Input: dimensioned drawing with shaded views. Units: mm. Origin: part minimum x, y, z. A direction names the side the tool comes from. Round coordinates to 2 decimals unless told otherwise and drop trailing zeros. Write each loop counter-clockwise with the first axis right and the second up, starting at its lowest first coordinate (ties: lowest second). Pieces come first, ordered by that corner, then holes. Notation, with made-up numbers: M 87,-34.5 L 102,-34.5 A29 ccw 102,-5.5 Z; hole C -36,11.5 d4. An arc over 180 degrees is marked long. Answer in a Markdown table with one row per item. Add a question column.
Item 1: Contact query for flat-ended pins moving along their axis: pin 1 (12 mm diameter, centred on x = 569, z = 661.5, fed in from -Y); pin 2 (12 mm diameter, centred on y = 489, z = 665.5, fed in from +X). Output: stop coordinate, or through.
Item 2: Cut plane D-D on z = 83. Return loops of the section in (x, y), and give its area (3 significant figures).
Item 3: Set-up query: the marked faces 1, 2, 3 and 4. Return all of +Z, -Z, +X, -X, +Y, -Y with unobstructed straight access to the full face (end or side cutting, diameter ignored); none if empty.
Item 4: Cut plane A-A on y = 268. Return loops of the section in (x, z) (1 decimal).
Item 5: Material intervals for probe 1 along Z at (x, y) = (132, 424.5) (1 decimal); probe 2 along Y at (x, z) = (1610, 397.5); probe 3 along X at (y, z) = (741, 596.5), sorted ascending.
Item 6: Cut plane B-B on x = 141.5. Return loops of the section in (y, z) (1 decimal).
Item 7: Cut plane C-C on y = 79. Return loops of the section in (x, z) (1 decimal), and give its area (3 significant figures).
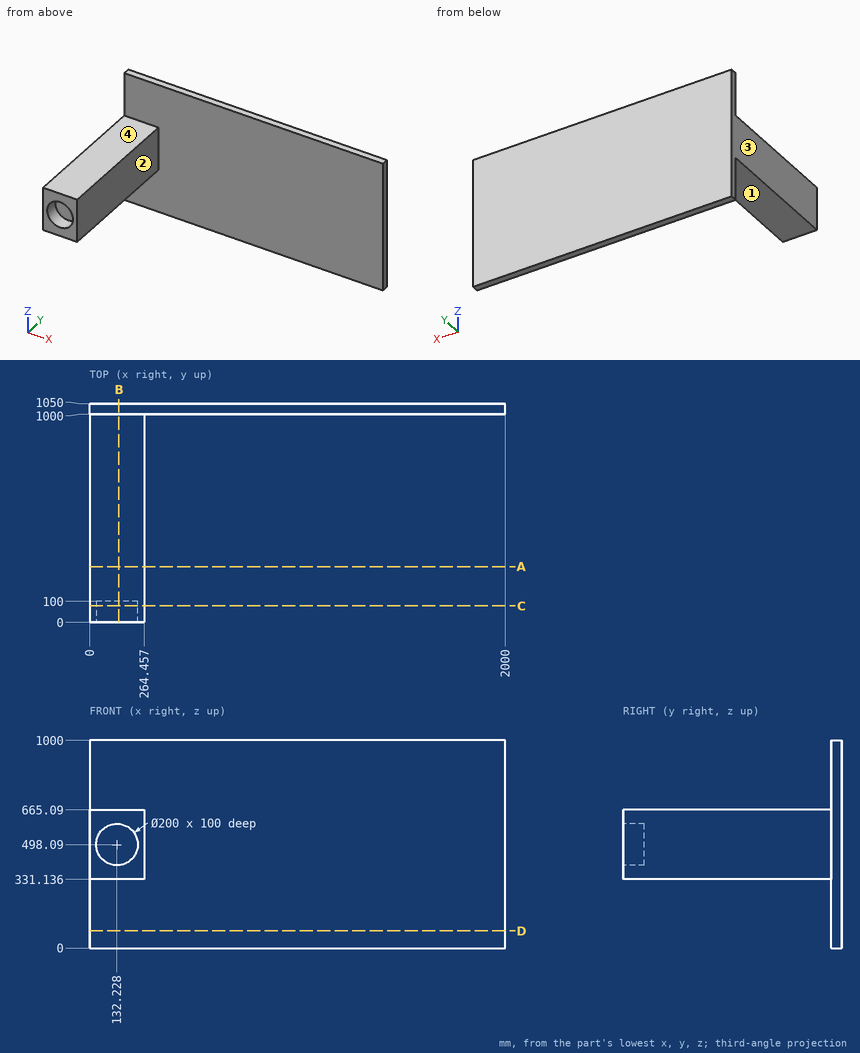
Results below:
| question | item | result |
|---|---|---|
| 1 | pin 1 | y = 1000 |
| 1 | pin 2 | x = 264.46 |
| 2 | outline | M 0,1000 L 2000,1000 L 2000,1050 L 0,1050 Z |
| 2 | area | 100,000 mm2 |
| 3 | face 1 | -Z, +X, -X, -Y |
| 3 | face 2 | +Z, -Z, +X, -Y |
| 3 | face 3 | +Z, -Z, -X, +Y, -Y |
| 3 | face 4 | +Z, +X, -X, -Y |
| 4 | outline | M 0,331.1 L 264.5,331.1 L 264.5,665.1 L 0,665.1 Z |
| 5 | probe 1 | 331.1 to 665.1 |
| 5 | probe 2 | 1000 to 1050 |
| 5 | probe 3 | 0 to 264.46 |
| 6 | outline | M 0,331.1 L 1000,331.1 L 1000,0 L 1050,0 L 1050,1000 L 1000,1000 L 1000,665.1 L 0,665.1 L 0,597.7 L 100,597.7 L 100,398.5 L 0,398.5 Z |
| 7 | outline | M 0,331.1 L 264.5,331.1 L 264.5,665.1 L 0,665.1 Z; hole C 132.2,498.1 d200 |
| 7 | area | 56,900 mm2 |
